from build123d import *

# Parameters (mm, degrees)
EXTRUDE_2_DEPTH     = 170
SKETCH_5_W          = 160
SKETCH_5_H          = 60
CUT_EXTRUDE_2_DEPTH = 10
SKETCH_6_W          = 160
SKETCH_6_H          = 10
CUT_EXTRUDE_3_DEPTH = 10
SKETCH_7_W          = 160
SKETCH_7_H          = 55
CUT_EXTRUDE_4_DEPTH = 5
SKETCH_8_W          = 160
SKETCH_8_H          = 10
CUT_EXTRUDE_5_DEPTH = 5
CUT_EXTRUDE_6_DEPTH = 5


with BuildPart() as part:
    # 草图1 → 凸台-拉伸2 (new body)
    with BuildSketch(Plane(origin=(0, 0, 0), x_dir=(0, 0, -1), z_dir=(1, 0, 0))):
        Polygon((0, 0), (15, 0), (20, 0), (80, 0), (80, 10), (20, 10), (15, 10), (5, 10), (5, 70), (-15, 70), (-15, 65), (0, 65), align=None)
    extrude(amount=EXTRUDE_2_DEPTH)

    # 草图5 → 切除-拉伸2 (cut)
    with BuildSketch(Plane(origin=(0, 10, 0), x_dir=(1, 0, 0), z_dir=(0, 1, 0))):
        with Locations((85, 50)):
            Rectangle(SKETCH_5_W, SKETCH_5_H)
    extrude(amount=-CUT_EXTRUDE_2_DEPTH, mode=Mode.SUBTRACT)

    # 草图6 → 切除-拉伸3 (cut)
    with BuildSketch(Plane(origin=(0, 10, 0), x_dir=(1, 0, 0), z_dir=(0, 1, 0))):
        with Locations((85, 10)):
            Rectangle(SKETCH_6_W, SKETCH_6_H)
    extrude(amount=-CUT_EXTRUDE_3_DEPTH, mode=Mode.SUBTRACT)

    # 草图7 → 切除-拉伸4 (cut)
    with BuildSketch(Plane(origin=(0, 0, -5), x_dir=(-1, 0, 0), z_dir=(0, 0, -1))):
        with Locations((-85, 37.5)):
            Rectangle(SKETCH_7_W, SKETCH_7_H)
    extrude(amount=-CUT_EXTRUDE_4_DEPTH, mode=Mode.SUBTRACT)

    # 草图8 → 切除-拉伸5 (cut)
    with BuildSketch(Plane(origin=(0, 0, -5), x_dir=(-1, 0, 0), z_dir=(0, 0, -1))):
        with Locations((-85, 5)):
            Rectangle(SKETCH_8_W, SKETCH_8_H)
    extrude(amount=-CUT_EXTRUDE_5_DEPTH, mode=Mode.SUBTRACT)

    # 草图9 → 切除-拉伸6 (cut)
    with BuildSketch(Plane(origin=(0, 70, 0), x_dir=(1, 0, 0), z_dir=(0, 1, 0))):
        Polygon((85, -15), (105, -15), (105, -2), (65, -2), (65, -15), align=None)
    extrude(amount=-CUT_EXTRUDE_6_DEPTH, mode=Mode.SUBTRACT)


solid = part.part
Design review of the part built by this model. Coordinates are the model's own, in mm. A direction names the side the tool comes from. Give positions to 0.01 mm unless a question says otherwise; leave off trailing zeros. Write each loop counter-clockwise with the first axis right and the second up, starting at its lowest first coordinate (ties: lowest second). Pieces come first, ordered by that corner, then holes. Notation, with made-up numbers: M 23,21.5 L 37,21.5 A10 cw 37,33.5 Z; hole C 88.25,6 d11. An arc over 180 degrees is marked long. Return JSON: item names as keys, results as strings. Group by question number.
Item 1: Wall thickness on line 1 along X through (y, z) = (9, -52); line 2 along Y through (x, z) = (46.5, 4); line 3 along Z through (x, y) = (113, 6.5): over which ranges is each line inside the solid? List them lowest first.
Item 2: Tool access review of faces 5 (the flat face through (5, 26, -4)), 6 (the flat face through (84, 5, -15)), 7 (the flat face through (85, 10, -18)): name each direction out of +Z, -Z, +X, -X, +Y, -Y from which nothing blocks a thin tool from reaching the whole face with its end or side.
Item 3: The part is to be moulded in two halves that separate along X. For faces 1 (the flat face through (84, 70, 0)), 2 (the flat face through (65, 68, 8)), 3 (the flat face through (84, 5, -20)), 4 (the flat face through (170, 9, -22)), say which applies: pulls with the +X half, pulls with the -X half, needs draft (parallel to the pull), parting line crosses it, or undercut.
Item 4: Clearance check with flat-ended pins moving along their axes: pin 1 Ø1.5 at (x, y) = (168, 25) entering from +Z; pin 2 Ø7.5 at (y, z) = (23, -11) entering from -X; pin 3 Ø2.5 at (x, y) = (82.5, 67.5) entering from +Z; pin 4 Ø11 at (x, y) = (100.5, 3) entering from -Z. State where each tip first meets the part, or that it passes through.
Item 5: Take a section at A-A (x = 67.5). Give the boundary of the cut face in (y, z), plus the area to 3 significant figures.
Item 6: Take a section at C-C (y = 7.5). Give the boundary of the cut face in (x, z), plus the area to 3 significant figures.
Item 7: Take a section at B-B (z = -71). Give the boundary of the cut face in (x, y), plus the area to 3 significant figures.
Return value:
{
 "1": {"line 1": "x = 0 to 5, 165 to 170", "line 2": "y = 65 to 70", "line 3": "z = -20 to -15"},
 "2": {"face 5": "+Z, -Y", "face 6": "+Z, +Y, -Y", "face 7": "-Z, +X, -X, +Y"},
 "3": {"face 1": "needs draft", "face 2": "undercut", "face 3": "undercut", "face 4": "pulls with the +X half"},
 "4": {"pin 1": "stops at z = 0", "pin 2": "passes through", "pin 3": "stops at z = 2", "pin 4": "stops at z = -20"},
 "5": {"outline": "M 0,-20 L 10,-20 L 10,-15 L 0,-15 Z; M 65,-5 L 70,-5 L 70,2 L 65,2 Z", "area": "85.0 mm2"},
 "6": {"outline": "M 0,-80 L 5,-80 L 5,-20 L 165,-20 L 165,-80 L 170,-80 L 170,0 L 165,0 L 165,-15 L 5,-15 L 5,0 L 0,0 Z", "area": "1,600 mm2"},
 "7": {"outline": "M 0,0 L 5,0 L 5,10 L 0,10 Z; M 165,0 L 170,0 L 170,10 L 165,10 Z", "area": "100 mm2"}
}
